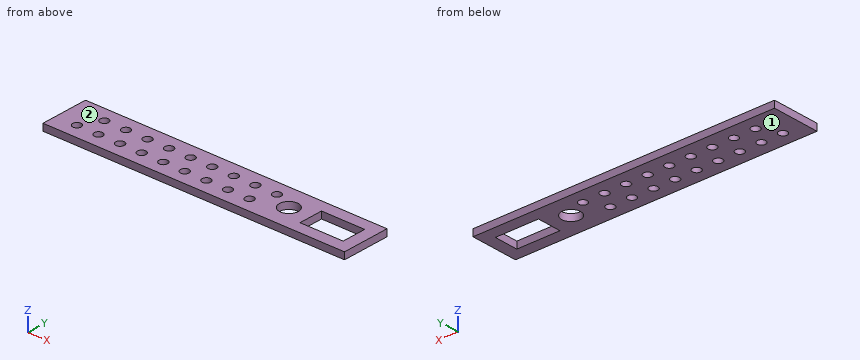
from build123d import *

# Parameters (mm, degrees)
SKETCH_R   = 7.9375
SKETCH_R_2 = 17.5
SKETCH_W   = 80
SKETCH_H   = 45
PAD_DEPTH  = 12.7


with BuildPart() as part:
    # Sketch → Pad (new body)
    with BuildSketch(Plane.XY):
        Polygon((0, 88.9), (540, 88.9), (540, 0), (0, 0), (-19.05, 0), (-19.05, 88.9), align=None)
        with Locations((20, 27.01875)):
            Circle(SKETCH_R, mode=Mode.SUBTRACT)
        with Locations((60, 27.01875)):
            Circle(SKETCH_R, mode=Mode.SUBTRACT)
        with Locations((397.5, 44.45)):
            Circle(SKETCH_R_2, mode=Mode.SUBTRACT)
        with Locations((478.05, 44.45)):
            Rectangle(SKETCH_W, SKETCH_H, mode=Mode.SUBTRACT)
        with Locations((40, 61.88125)):
            Circle(SKETCH_R, mode=Mode.SUBTRACT)
        with Locations((100, 27.01875)):
            Circle(SKETCH_R, mode=Mode.SUBTRACT)
        with Locations((140, 27.01875)):
            Circle(SKETCH_R, mode=Mode.SUBTRACT)
        with Locations((180, 27.01875)):
            Circle(SKETCH_R, mode=Mode.SUBTRACT)
        with Locations((220, 27.01875)):
            Circle(SKETCH_R, mode=Mode.SUBTRACT)
        with Locations((260, 27.01875)):
            Circle(SKETCH_R, mode=Mode.SUBTRACT)
        with Locations((300, 27.01875)):
            Circle(SKETCH_R, mode=Mode.SUBTRACT)
        with Locations((340, 27.01875)):
            Circle(SKETCH_R, mode=Mode.SUBTRACT)
        with Locations((80, 61.88125)):
            Circle(SKETCH_R, mode=Mode.SUBTRACT)
        with Locations((120, 61.88125)):
            Circle(SKETCH_R, mode=Mode.SUBTRACT)
        with Locations((160, 61.88125)):
            Circle(SKETCH_R, mode=Mode.SUBTRACT)
        with Locations((200, 61.88125)):
            Circle(SKETCH_R, mode=Mode.SUBTRACT)
        with Locations((240, 61.88125)):
            Circle(SKETCH_R, mode=Mode.SUBTRACT)
        with Locations((280, 61.88125)):
            Circle(SKETCH_R, mode=Mode.SUBTRACT)
        with Locations((320, 61.88125)):
            Circle(SKETCH_R, mode=Mode.SUBTRACT)
        with Locations((360, 61.88125)):
            Circle(SKETCH_R, mode=Mode.SUBTRACT)
    extrude(amount=PAD_DEPTH)


solid = part.part
Check sheet for the modelled part. Datum: model origin and axes. Units: mm. Face numbers are marked on the shaded views. Round coordinates to 2 decimals unless told otherwise and drop trailing zeros. Order: outer loops, then holes, each group sorted by start corner. A loop starts at its lowest first (then second) coordinate and runs counter-clockwise, first axis right, second up.
(1) Cross-section at B-B, the plane z = 9.25. State how many separate pieces and enclosed holes the cut face has, and give its area (3 significant figures).
(2) Scan lines: probe 1 along X at (y, z) = (46, 3.75); probe 2 along X at (y, z) = (50.5, 11.75); probe 3 along Y at (x, z) = (80, 8). Record each from-to range of solid material in increasing order.
(3) Cross-section at A-A, the plane x = 455.5. Enter the section's corners in (y, z).
(4) Draft check along Z on the marked faces 1 and 2. Enter one of: pulls with the +Z half, pulls with the -Z half, needs draft (parallel to the pull), parting line crosses it, or undercut.
(5) Cross-section at C-C, the plane x = 200. Enter the section's corners in (y, z), and give its area (3 significant figures).
Check sheet entries:
1. separate pieces: 1
1. enclosed holes: 20
1. area: 41,600 mm2
2. probe 1: x = -19.05 to 380.07, 414.93 to 438.05, 518.05 to 540
2. probe 2: x = -19.05 to 381.08, 413.92 to 438.05, 518.05 to 540
2. probe 3: y = 0 to 53.94, 69.82 to 88.9
3. outline: (0, 0) - (21.95, 0) - (21.95, 12.7) - (0, 12.7) - close; (66.95, 0) - (88.9, 0) - (88.9, 12.7) - (66.95, 12.7) - close
4. face 1: pulls with the -Z half
4. face 2: pulls with the +Z half
5. outline: (0, 0) - (53.94, 0) - (53.94, 12.7) - (0, 12.7) - close; (69.82, 0) - (88.9, 0) - (88.9, 12.7) - (69.82, 12.7) - close
5. area: 927 mm2
